```python
from build123d import *

# Parameters (mm, degrees)
ESQUISSE1_R        = 14
BOSS_EXTRU_1_DEPTH = 14
ESQUISSE2_R        = 10.5
BOSS_EXTRU_2_DEPTH = 2
ESQUISSE4_R        = 20
BOSS_EXTRU_3_DEPTH = 4
ESQUISSE5_R        = 20
BOSS_EXTRU_4_DEPTH = 2
CHANFREIN1_SIZE    = 2
CHANFREIN1_SIZE2   = 1.154700538


with BuildPart() as part:
    # Esquisse1 → Boss.-Extru.1 (new body)
    with BuildSketch(Plane(origin=(0, 0, 0), x_dir=(1, 0, 0), z_dir=(0, 1, 0))):
        with Locations(Location((0, 0, 0), (0, 0, 270))):
            Circle(ESQUISSE1_R)
    extrude(amount=BOSS_EXTRU_1_DEPTH)

    # Esquisse2 → Boss.-Extru.2 (add)
    with BuildSketch(Plane(origin=(0, 14, 0), x_dir=(1, 0, 0), z_dir=(0, 1, 0))):
        with Locations(Location((0, 0, 0), (0, 0, 270))):
            Circle(ESQUISSE2_R)
    extrude(amount=BOSS_EXTRU_2_DEPTH)

    # Esquisse4 → Boss.-Extru.3 (add)
    with BuildSketch(Plane(origin=(0, 16, 0), x_dir=(1, 0, 0), z_dir=(0, 1, 0))):
        with Locations(Location((0, 0, 0), (0, 0, 270))):
            Circle(ESQUISSE4_R)
    extrude(amount=BOSS_EXTRU_3_DEPTH)

    # Esquisse5 → Boss.-Extru.4 (add)
    with BuildSketch(Plane(origin=(0, 20, 0), x_dir=(1, 0, 0), z_dir=(0, 1, 0))):
        with Locations(Location((0, 0, 0), (0, 0, 270))):
            Circle(ESQUISSE5_R)
    extrude(amount=BOSS_EXTRU_4_DEPTH)

    # Chanfrein1
    chanfrein1_edges = [part.edges().sort_by_distance(p)[0] for p in [
        (0, 22, -20),
    ]]
    chanfrein1_side = [part.faces().sort_by_distance(p)[0] for p in [
        (0, 19, -20),
    ]]
    chamfer(chanfrein1_edges, length=CHANFREIN1_SIZE, length2=CHANFREIN1_SIZE2, reference=chanfrein1_side[0])


solid = part.part
```
Could you check a few things on this model? Use its own coordinates, in mm. A direction names the side the tool comes from. Coordinates: 2 decimals unless noted, no trailing zeros. Order: outer loops, then holes, each group sorted by start corner. A loop starts at its lowest first (then second) coordinate and runs counter-clockwise, first axis right, second up. Notation, with made-up numbers: M 21.5,33 L 61.5,33 A34 ccw 61.5,65 Z; hole C 60.5,-15.75 d4. An arc over 180 degrees is marked long. Use a Markdown table: item, result. Add a question column.
Q1. Which directions (+Z, -Z, +X, -X, +Y, -Y) give clear straight access to the entire face, cutting with the end or side of a thin tool? Please do faces 4 (the flat face through (0, 22, 0)), 5 (the cylindrical face through (-13.67, 6.9, -3.03)), 6 (the cylindrical face through (3.2, 15, 10)).
Q2. I want a section at B-B on x = 0. List the corners of the cut face in (y, z) for me, then the cut area to 3 significant figures.
Q3. I want a section at C-C on y = 16.75. List the corners of the cut face in (x, z) for me.
Q4. We'd pull the mould along Y, two halves only. Please class faces 1 (the cylindrical face through (-19.524, 17.972, -4.336)), 2 (the flat face through (9.4, 14, 5.1)), 3 (the flat face through (0, 0, 0)): pulls with the +Y half, pulls with the -Y half, needs draft (parallel to the pull), parting line crosses it, or undercut.
Q5. If I drill on L1, parallel to Y at x = 13, z = 3.5; L2, parallel to Y at x = -14.5, z = 6.5; L3, parallel to Z at x = -2.5, y = 10, over which ranges is the centre line in solid material (lowest first)?
Q6. I'm going to push flat-ended pins straight in: pin 1 (2 mm diameter, centred on x = 2, y = 18, fed in from -Z) (3 decimals); pin 2 (1 mm diameter, centred on y = 10.5, z = 7.5, fed in from +X); pin 3 (2 mm diameter, centred on x = 2.5, y = 2.5, fed in from -Z). Where does each tip first touch, or does it pass through?
Q7. I want a section at A-A on z = 0. List the corners of the cut face in (x, y) for me.
Q8. I want a section at D-D on y = 13.25. List the corners of the cut face in (x, z) for me.
Checked values:
| question | item | result |
|---|---|---|
| 1 | face 4 | +Z, -Z, +X, -X, +Y |
| 1 | face 5 | -Y |
| 1 | face 6 | none |
| 2 | outline | M 0,-14 L 14,-14 L 14,-10.5 L 16,-10.5 L 16,-20 L 20,-20 L 22,-18.85 L 22,18.85 L 20,20 L 16,20 L 16,10.5 L 14,10.5 L 14,14 L 0,14 Z |
| 2 | area | 672 mm² |
| 3 | outline | C 0,0 d40 |
| 4 | face 1 | needs draft |
| 4 | face 2 | undercut |
| 4 | face 3 | pulls with the -Y half |
| 5 | L1 | 0 to 14, 16 to 22 |
| 5 | L2 | 16 to 22 |
| 5 | L3 | -13.77 to 13.77 |
| 6 | pin 1 | z = -19.975 |
| 6 | pin 2 | x = 12.12 |
| 6 | pin 3 | z = -13.92 |
| 7 | outline | M -20,16 L -10.5,16 L -10.5,14 L -14,14 L -14,0 L 14,0 L 14,14 L 10.5,14 L 10.5,16 L 20,16 L 20,20 L 18.85,22 L -18.85,22 L -20,20 Z |
| 8 | outline | C 0,0 d28 |
